Design review of the part shown in the three views and the two pictorial views. Dimensions are in mm from the part's minimum x, y and z. Give positions to 0.01 mm unless a question says otherwise; leave off trailing zeros. Loops run counter-clockwise (first coordinate to the right, second up) from the corner with the lowest first, then second, coordinate; pieces in that order, holes last. Notation, with made-up numbers: (-0.5, 14) - (44.5, 14) arc R27 ccw to (44.5, 30) - close; hole circle Ø5 at (-15.75, 89.5). An arc over 180 degrees is marked (long way). Answer in a Markdown table with one row per item.
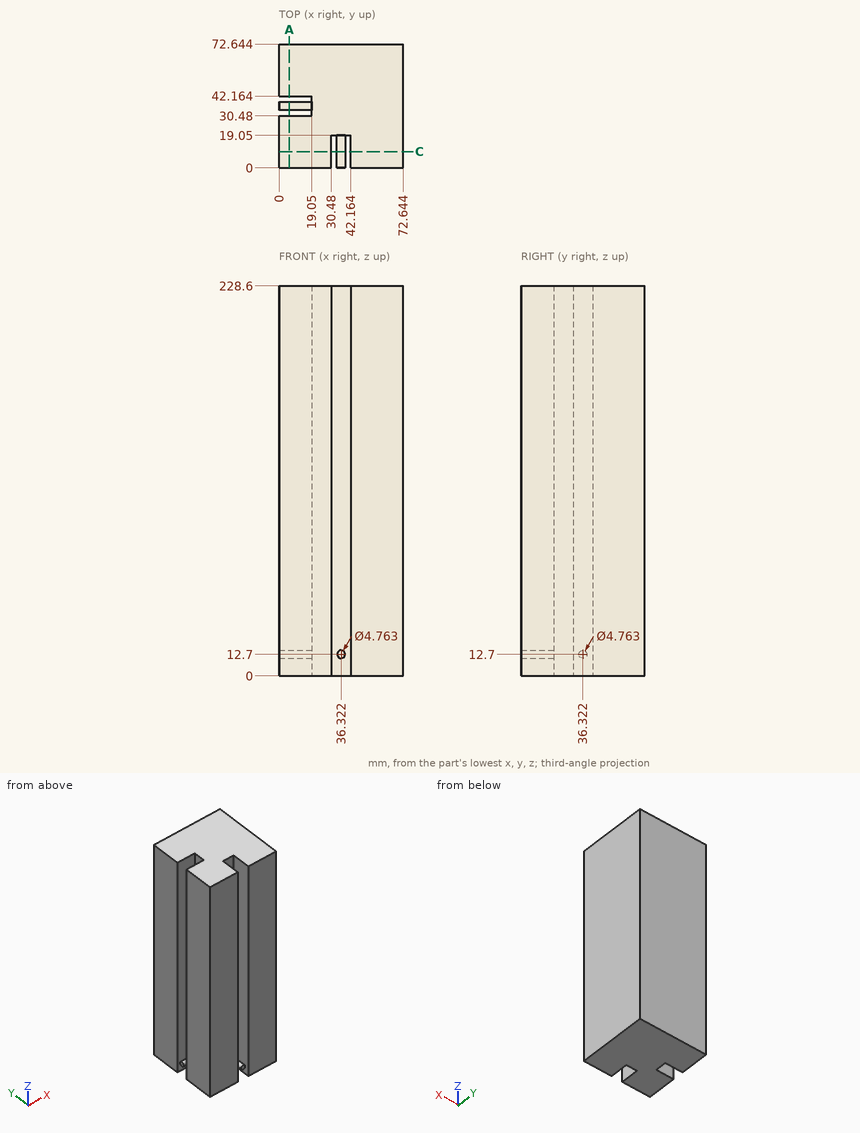
1. We need section A-A, the plane x = 6. Give the boundary of the cut face in (y, z) (1 decimal).
Values:
| item | result |
|---|---|
| outline | (0, 0) - (30.5, 0) - (30.5, 228.6) - (0, 228.6) - close; circle Ø4.8 at (36.3, 12.7); (42.2, 0) - (72.6, 0) - (72.6, 228.6) - (42.2, 228.6) - close |
2. Wall thickness on line 1 (X direction, y = 15.5, z = 56) (1 decimal): over which ranges is the line inside the solid? List them lowest first. Write a range as [from, to].
Values:
| item | result |
|---|---|
| line 1 | x = [0, 30.5], [42.2, 72.6] |
3. Clearance check with flat-ended pins moving along their axes: pin 1 (13 mm diameter, centred on y = 39, z = 113.5, fed in from -X); pin 2 (2 mm diameter, centred on x = 38, z = 192, fed in from -Y). State where each tip first meets the part, or that it passes through.
Values:
| item | result |
|---|---|
| pin 1 | stops at x = 0 |
| pin 2 | stops at y = 19.05 |
